Part model, mm, in its own coordinate system. Face numbers are marked on the shaded views. A direction names the side the tool comes from. Round coordinates to 2 decimals unless told otherwise and drop trailing zeros. Loops run counter-clockwise (first coordinate to the right, second up) from the corner with the lowest first, then second, coordinate; pieces in that order, holes last. Notation, with made-up numbers: (-19.75, 64.25) -> (35.25, 64.25) arc R21 ccw to (35.25, 85.25) -> close; hole circle Ø1 at (89, 48.5). An arc over 180 degrees is marked (long way). Use a Markdown table: item, result. Add a question column.
Item 1: Cut at A-A, the plane x = 15.5. List the corners of the cut face in (y, z), plus the area to 3 significant figures.
Item 2: Flat gauge pins, fed straight in: pin 1 (4 mm diameter, centred on x = 32, z = 31, fed in from +Y); pin 2 (3.5 mm diameter, centred on y = 2, z = 17.5, fed in from -X); pin 3 (12 mm diameter, centred on y = 21.5, z = 14, fed in from +X). Where does each tip first touch, or does it go through?
Item 3: Cut at B-B, the plane z = 26. List the corners of the cut face in (x, y), plus the area to 3 significant figures.
Item 4: Probe line 1 (Z direction, x = 37.1, y = 9); line 2 (X direction, y = 23.5, z = 38); line 3 (Y direction, x = 37.65, z = 40). List the from-to ranges inside material, lowest first. Write a range as [from, to].
Item 5: Two-plate mould, pull along X, no slides. Class the marked faces 4, 5 and 6: pulls with the +X half, pulls with the -X half, needs draft (parallel to the pull), parting line crosses it, or undercut.
Item 6: Which spindle directions (+Z, -Z, +X, -X, +Y, -Y) get a long thin tool onto all of the face, cutting with end or side? Do the marked faces 1, 2 and 3. Say none if no direction does.
Item 7: Cut at D-D, the plane y = 5. List the corners of the cut face in (x, z).
Item 8: Cut at C-C, the plane y = 9. List the corners of the cut face in (x, z), plus the area to 3 significant figures.
```python
from build123d import *

# Parameters (mm, degrees)
EXTRUDE_1_DEPTH        = 42
SKETCH_2_R             = 2.5
SKETCH_2_R_2           = 5
CUT_EXTRUDE_1_DEPTH    = 57.329388422
EXTRUDE_2_DEPTH        = 18
SKETCH_5_R             = 4
CUT_EXTRUDE_2_DEPTH    = 61.704200843
HOLE_WIZARD_M3_1_D     = 2.5
HOLE_WIZARD_M3_1_DEPTH = 7.5
HOLE_WIZARD_M3_1_TIP   = 0.751075774
SKETCH_9_W             = 22
SKETCH_9_H             = 4
CUT_EXTRUDE_4_DEPTH    = 61.761830124
FILLET_1_R             = 2
SKETCH_10_W            = 10
SKETCH_10_H            = 24
CUT_EXTRUDE_5_DEPTH    = 61.761830124
FILLET_2_R             = 2
SKETCH_11_W            = 4
SKETCH_11_H            = 14
CUT_EXTRUDE_8_DEPTH    = 62.911226769
FILLET_3_R             = 2
SKETCH_12_W            = 28
SKETCH_12_H            = 14
CUT_EXTRUDE_9_DEPTH    = 22
HOLE_WIZARD_M2_1_D     = 1.6
HOLE_WIZARD_M2_1_DEPTH = 4
HOLE_WIZARD_M2_1_TIP   = 0.480688495
CHAMFER_1_SIZE         = 1


with BuildPart() as part:
    # 草图1 → 凸台-拉伸1 (new body)
    with BuildSketch(Plane.XY):
        Polygon((0, 0), (0, 25), (3, 25), (3, 3), (25, 3), (25, 25), (28, 25), (28, 0), align=None)
    extrude(amount=EXTRUDE_1_DEPTH)

    # 草图2 → 切除-拉伸1 (cut, through all)
    with BuildSketch(Plane(origin=(28, 0, 0), x_dir=(0, 0, -1), z_dir=(1, 0, 0))):
        with Locations(Location((-5, 16, 0), (0, 0, 90))):
            Circle(SKETCH_2_R)
        with Locations(Location((-33, 16, 0), (0, 0, 90))):
            Circle(SKETCH_2_R_2)
    extrude(amount=-CUT_EXTRUDE_1_DEPTH, mode=Mode.SUBTRACT)

    # 草图3 → 凸台-拉伸2 (add)
    with BuildSketch(Plane.XY.offset(42)):
        Polygon((28, 0), (38, 0), (38, 25), (36, 25), (36, 3), (28, 3), align=None)
    extrude(amount=-EXTRUDE_2_DEPTH)

    # 草图5 → 切除-拉伸2 (cut, through all)
    with BuildSketch(Plane.ZY.offset(-36)):
        with Locations((33, 16)):
            Circle(SKETCH_5_R)
    extrude(amount=-CUT_EXTRUDE_2_DEPTH, mode=Mode.SUBTRACT)

    # M3 螺纹孔1
    with Locations(Plane(origin=(20, 3, 3), x_dir=(0, 0, 1), z_dir=(0, 1, 0))):
        with Locations((0, 0), (0, -12), (32, 0), (32, -12)):
            Hole(HOLE_WIZARD_M3_1_D / 2, depth=HOLE_WIZARD_M3_1_DEPTH)
            with Locations((0, 0, -(HOLE_WIZARD_M3_1_DEPTH + HOLE_WIZARD_M3_1_TIP / 2))):  # 118° drill point
                Cone(0, HOLE_WIZARD_M3_1_D / 2, HOLE_WIZARD_M3_1_TIP, mode=Mode.SUBTRACT)

    # 草图9 → 切除-拉伸4 (cut, through all)
    with BuildSketch(Plane(origin=(0, 3, 0), x_dir=(1, 0, 0), z_dir=(0, 1, 0))):
        with Locations((14, -40)):
            Rectangle(SKETCH_9_W, SKETCH_9_H)
    extrude(amount=-CUT_EXTRUDE_4_DEPTH, mode=Mode.SUBTRACT)

    # 圆角1
    fillet_1_edges = [part.edges().sort_by_distance(p)[0] for p in [
        (3, 1.5, 38),
        (25, 1.5, 38),
    ]]
    fillet(fillet_1_edges, radius=FILLET_1_R)

    # 草图10 → 切除-拉伸5 (cut, through all)
    with BuildSketch(Plane(origin=(0, 3, 0), x_dir=(1, 0, 0), z_dir=(0, 1, 0))):
        with Locations((14, -19)):
            Rectangle(SKETCH_10_W, SKETCH_10_H)
    extrude(amount=-CUT_EXTRUDE_5_DEPTH, mode=Mode.SUBTRACT)

    # 圆角2
    fillet_2_edges = [part.edges().sort_by_distance(p)[0] for p in [
        (19, 1.5, 7),
        (19, 1.5, 31),
        (9, 1.5, 31),
        (9, 1.5, 7),
    ]]
    fillet(fillet_2_edges, radius=FILLET_2_R)

    # 草图11 → 切除-拉伸8 (cut, through all)
    with BuildSketch(Plane(origin=(0, 25, 0), x_dir=(1, 0, 0), z_dir=(0, 1, 0))):
        with Locations((26, -17)):
            Rectangle(SKETCH_11_W, SKETCH_11_H)
        with Locations((2, -17)):
            Rectangle(SKETCH_11_W, SKETCH_11_H)
    extrude(amount=-CUT_EXTRUDE_8_DEPTH, mode=Mode.SUBTRACT)

    # 圆角3
    fillet_3_edges = [part.edges().sort_by_distance(p)[0] for p in [
        (4, 1.5, 10),
        (4, 1.5, 24),
        (24, 1.5, 24),
        (24, 1.5, 10),
    ]]
    fillet(fillet_3_edges, radius=FILLET_3_R)

    # 草图12 → 切除-拉伸9 (cut)
    with BuildSketch(Plane(origin=(0, 25, 0), x_dir=(1, 0, 0), z_dir=(0, 1, 0))):
        with Locations((14, -17)):
            Rectangle(SKETCH_12_W, SKETCH_12_H)
    extrude(amount=-CUT_EXTRUDE_9_DEPTH, mode=Mode.SUBTRACT)

    # M2 螺纹孔1
    with Locations(Plane(origin=(38, 23, 40), x_dir=(0, 0, 1), z_dir=(1, 0, 0))):
        with Locations((0, 0), (-14, 0), (-14, 14), (0, 14)):
            Hole(HOLE_WIZARD_M2_1_D / 2, depth=HOLE_WIZARD_M2_1_DEPTH)
            with Locations((0, 0, -(HOLE_WIZARD_M2_1_DEPTH + HOLE_WIZARD_M2_1_TIP / 2))):  # 118° drill point
                Cone(0, HOLE_WIZARD_M2_1_D / 2, HOLE_WIZARD_M2_1_TIP, mode=Mode.SUBTRACT)

    # 倒角1
    chamfer_1_edges = [part.edges().sort_by_distance(p)[0] for p in [
        (26.5, 25, 42),
        (26.5, 25, 10),
        (1.5, 25, 24),
        (1.5, 25, 10),
        (26.5, 25, 24),
        (1.5, 25, 42),
        (37, 25, 24),
        (37, 25, 42),
        (1.5, 25, 0),
        (26.5, 25, 0),
    ]]
    chamfer(chamfer_1_edges, length=CHAMFER_1_SIZE)


solid = part.part
```
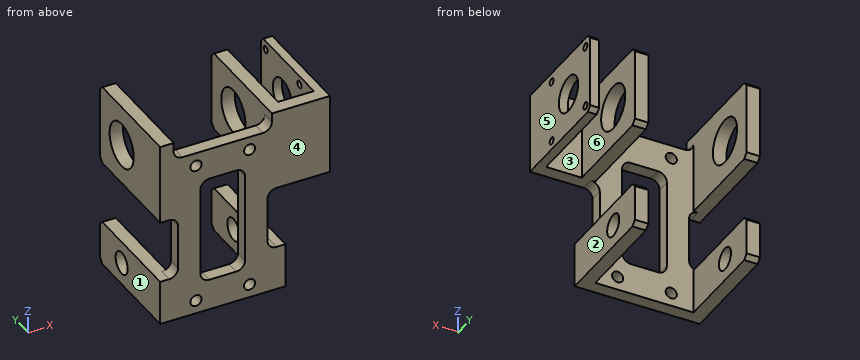
A:
| question | item | result |
|---|---|---|
| 1 | outline | (0, 0) -> (3, 0) -> (3, 7) -> (0, 7) -> close; (0, 31) -> (3, 31) -> (3, 38) -> (0, 38) -> close |
| 1 | area | 42.0 mm^2 |
| 2 | pin 1 | stops at y = 3 |
| 2 | pin 2 | stops at x = 4 |
| 2 | pin 3 | stops at x = 28 |
| 3 | outline | (0, 0) -> (9, 0) -> (9, 3) -> (3, 3) -> (3, 25) -> (0, 25) -> close; (19, 0) -> (38, 0) -> (38, 8.2) -> (36, 8.2) -> (36, 3) -> (28, 3) -> (28, 25) -> (25, 25) -> (25, 3) -> (19, 3) -> close; (36, 9.8) -> (38, 9.8) -> (38, 22.2) -> (36, 22.2) -> close; (36, 23.8) -> (38, 23.8) -> (38, 25) -> (36, 25) -> close |
| 3 | area | 254 mm^2 |
| 4 | line 1 | z = [24, 25.2], [26.8, 39.2], [40.8, 42] |
| 4 | line 2 | x = [0, 3], [25, 28], [36, 38] |
| 4 | line 3 | y = [0, 8.2], [9.8, 22.2], [23.8, 25] |
| 5 | face 4 | needs draft |
| 5 | face 5 | pulls with the +X half |
| 5 | face 6 | undercut |
| 6 | face 1 | +Z, -Z, -X, +Y, -Y |
| 6 | face 2 | -Z, +X, +Y, -Y |
| 6 | face 3 | +Z, -Z, +Y |
| 7 | outline | (0, 0) -> (3, 0) -> (3, 10) -> (0, 10) -> close; (0, 24) -> (3, 24) -> (3, 42) -> (0, 42) -> close; (25, 0) -> (28, 0) -> (28, 10) -> (25, 10) -> close; (25, 24) -> (28, 24) -> (28, 42) -> (25, 42) -> close; (36, 24) -> (38, 24) -> (38, 42) -> (36, 42) -> close |
| 8 | outline | (0, 0) -> (3, 0) -> (3, 10) -> (0, 10) -> close; (0, 24) -> (3, 24) -> (3, 42) -> (0, 42) -> close; (25, 0) -> (28, 0) -> (28, 10) -> (25, 10) -> close; (25, 24) -> (28, 24) -> (28, 42) -> (25, 42) -> close; (36, 24) -> (38, 24) -> (38, 25.2) -> (36, 25.2) -> close; (36, 26.8) -> (38, 26.8) -> (38, 39.2) -> (36, 39.2) -> close; (36, 40.8) -> (38, 40.8) -> (38, 42) -> (36, 42) -> close |
| 8 | area | 198 mm^2 |
